Here's how the part is built. I have some questions about the finished solid (model axes, mm). A direction names the side the tool comes from. Round coordinates to 2 decimals unless told otherwise and drop trailing zeros. Order: outer loops, then holes, each group sorted by start corner. A loop starts at its lowest first (then second) coordinate and runs counter-clockwise, first axis right, second up. Notation, with made-up numbers: (88.5, 70) - (119.5, 70) arc R13 ccw to (119.5, 88) - close; hole circle Ø11 at (62.5, -34). An arc over 180 degrees is marked (long way). One line per item, written item: value.
from build123d import *

# Parameters (mm, degrees)
F1_DEPTH    = 63
F2_DEPTH    = 2.5
F3_T        = 4
F3_T3_DEPTH = 132.2533825366
F3_T5_DEPTH = 10.5
F3_T7_DEPTH = 71
F4_W        = 44
F4_H        = 52
F4_W_2      = 45
F5_DEPTH    = 4.5
F7_DEPTH    = 5
F9_DEPTH    = 25


# Not quite as in the source:
# - a shell that OpenCascade refuses in one call is made with other operations: the cavity is built on its own and cut out


with BuildPart() as f1:
    # F0 (on Top) → F1 (new body)
    with BuildSketch(Plane.XY):
        Polygon((26.2132732272, -24.0364130735), (26.2132732272, 29.9635869265), (-65.7867267728, 29.9635869265), (-65.7867267728, -100.0364130735), (26.2132732272, -69.0364130735), align=None)
        Polygon((158.2132732272, 65.9635869265), (26.2132732272, 65.9635869265), (26.2132732272, 29.9635869265), (26.2132732272, -24.0364130735), (26.2132732272, -69.0364130735), (40.4647773284, -64.234275822), (158.2132732272, -24.558152204), align=None)
    extrude(amount=F1_DEPTH)

    # F0 (on Top) → F2 (join)
    with BuildSketch(Plane.XY):
        Polygon((158.2132732272, 65.9635869265), (26.2132732272, 65.9635869265), (26.2132732272, 29.9635869265), (26.2132732272, -24.0364130735), (26.2132732272, -69.0364130735), (40.4647773284, -64.234275822), (158.2132732272, -24.558152204), align=None)
        Polygon((26.2132732272, -24.0364130735), (26.2132732272, 29.9635869265), (-65.7867267728, 29.9635869265), (-65.7867267728, -100.0364130735), (26.2132732272, -69.0364130735), align=None)
        Polygon((158.1303410754, -64.234275822), (158.2132732272, -24.558152204), (40.4647773284, -64.234275822), align=None)
    extrude(amount=F2_DEPTH)

    # F3: shell of thickness 4, made by hand


with BuildPart() as f3_core1:
    # F3_t2: copy of F1
    add(f1.part)

    # the walls: a layer under each face that stays
    f3_faces = [f3_core1.faces().sort_by_distance(p)[0] for p in [
        (46.2132732272, -62.2972826388, 31.5),
        (99.2975592019, -64.234275822, 1.25),
        (158.1718071513, -44.396214013, 1.25),
        (99.3390252778, -57.6215885524, 2.5),
        (158.2132732272, 20.7027173612, 31.5),
        (92.2132732272, 65.9635869265, 31.5),
        (26.2132732272, 47.9635869265, 31.5),
        (-19.7867267728, 29.9635869265, 31.5),
        (46.2132732272, -17.0364130735, 63),
        (-65.7867267728, -35.0364130735, 31.5),
    ]]
    thicken(f3_faces, amount=-F3_T, mode=Mode.SUBTRACT)

    # F3_s4 → F3_t3 (cut)
    with BuildSketch(Plane(origin=(13.1110220732, 4.4178443942, 0), x_dir=(0, 0, 1), z_dir=(0.9476482128, 0.3193162456, 0))):
        Polygon((2.54, 73.8325574618), (2.5, 69.7925574618), (-1.5, 69.7925574618), (-1.5, 73.7925574618), align=None)
    extrude(amount=F3_T3_DEPTH, mode=Mode.SUBTRACT)

    # F3_s6 → F3_t5 (cut)
    with BuildSketch(Plane.XY.offset(-4)):
        Polygon((40.4775499783, -64.3121817506), (39.1875123459, -60.4436829707), (39.8089787227, -60.234275822), (40.4647773284, -60.234275822), align=None)
    extrude(amount=F3_T5_DEPTH, mode=Mode.SUBTRACT)

    # F3_s8 → F3_t7 (cut)
    with BuildSketch(Plane.XY.offset(-4)):
        Polygon((26.1732732272, 30.0035869265), (30.2132732272, 29.9635869265), (30.2132732272, 25.9635869265), (26.2132732272, 25.9635869265), align=None)
    extrude(amount=F3_T7_DEPTH, mode=Mode.SUBTRACT)


with BuildPart() as f1_1:
    add(f1.part)

    # what is left inside the walls is the cavity
    f3_cavity = [f3_core1.part.solids().sort_by_distance(p)[0] for p in [
        (46.213273, -42.323879, 0.04),
    ]]
    add(f3_cavity, mode=Mode.SUBTRACT)

    # F4 (on face) → F5 (cut)
    with BuildSketch(Plane(origin=(-65.7867267728, 0, 0), x_dir=(0, -1, 0), z_dir=(-1, 0, 0))):
        with Locations((68.8298759162, 26)):
            Rectangle(F4_W, F4_H)
        with Locations((3.3298759162, 26)):
            Rectangle(F4_W_2, F4_H)
    extrude(amount=-F5_DEPTH, mode=Mode.SUBTRACT)

    # F6 (on face) → F7 (cut)
    with BuildSketch(Plane.YZ.offset(158.2132732272)):
        Polygon((36.0559523106, 44.5), (-11.5364130735, 44.5), (-11.5364130735, 0), (54.4635869265, 0), (54.4635869265, 44.5), align=None)
    extrude(amount=-F7_DEPTH, mode=Mode.SUBTRACT)

    # F8 (on face) → F9 (cut)
    with BuildSketch(Plane.XY.offset(2.5)):
        with BuildLine():
            ThreePointArc((107.1575140418, -54.484275822), (109.4556110807, -53.5323728609), (110.4075140418, -51.234275822))
            Line((110.4075140418, -51.234275822), (107.1575140418, -51.234275822))
            Line((107.1575140418, -51.234275822), (107.1575140418, -54.484275822))
        make_face()
        with BuildLine():
            Line((107.1575140418, -51.234275822), (110.4075140418, -51.234275822))
            ThreePointArc((110.4075140418, -51.234275822), (104.859417003, -48.9361787832), (107.1575140418, -54.484275822))
            Line((107.1575140418, -54.484275822), (107.1575140418, -51.234275822))
        make_face()
    extrude(amount=-F9_DEPTH, mode=Mode.SUBTRACT)


solid = f1_1.part
Q1. We'd pull the mould along X, two halves only. Please class faces 4 (the flat face through (30.213, 44, 29)), 5 (the flat face through (45, -16, 63)), 6 (the flat face through (26.213, 48, 31)): released by +X, released by -X, zero draft, split by the parting line, or undercut.
Results list:
face 4: undercut
face 5: zero draft
face 6: released by -X
Q2. If we section it at B-B, the plane y = -18: Please give me the cut outline in (x, z).
Results list:
outline: (-65.79, 52) - (-61.79, 52) - (-61.79, 59) - (154.21, 59) - (154.21, 0) - (158.21, 0) - (158.21, 63) - (-65.79, 63) - close
Q3. Which directions (+Z, -Z, +X, -X, +Y, -Y) give clear straight access to the entire face, cutting with the end or side of a thin tool? Please do faces 1 (the flat face through (-19, 29.964, 31)), 2 (the flat face through (125, -53, 2.5)), 3 (the flat face through (93, 61.964, 29)).
Results list:
face 1: +Z, -Z, -X, +Y
face 2: +Z, +X, -Y
face 3: -Z
Q4. If we section it at C-C, the plane z = 9: Please give me the cut outline in (x, y) (3 decimals), then the cut area to 3 significant figures.
Results list:
outline: (-65.787, -100.036) - (158.213, -24.558) - (158.213, -11.536) - (154.213, -11.536) - (154.213, -21.685) - (-61.787, -94.468) - (-61.787, -90.83) - (-65.787, -90.83) - close; (-65.787, -46.83) - (-61.787, -46.83) - (-61.787, -25.83) - (-65.787, -25.83) - close; (-65.787, 19.17) - (-61.787, 19.17) - (-61.787, 25.964) - (30.213, 25.964) - (30.213, 61.964) - (154.213, 61.964) - (154.213, 54.464) - (158.213, 54.464) - (158.213, 65.964) - (26.213, 65.964) - (26.213, 29.964) - (-65.787, 29.964) - close
area: 2,180 mm²
Q5. If I drill on line 1 along X through (y, z) = (48, 48); line 2 along X through (y, z) = (-13, 32); line 3 along Y through (x, z) = (15, 3.5), over which ranges is the centre line in solid material (lowest first)?
Results list:
line 1: 26.21 to 30.21, 154.21 to 158.21
line 2: 154.21 to 158.21
line 3: -72.81 to -68.59, 25.96 to 29.96
Q6. If we section it at D-D, the plane x = 145: Please give me the cut outline in (y, z), then the cut area to 3 significant figures.
Results list:
outline: (-64.23, 0) - (-24.79, 0) - (-24.79, 59) - (61.96, 59) - (61.96, 0) - (65.96, 0) - (65.96, 63) - (-29.01, 63) - (-29.01, 2.5) - (-64.23, 2.5) - close
area: 953 mm²
Q7. Will these pins go through, and if not, where does the flat tip stop? pin 1 (10 mm diameter, centred on x = 135.5, z = 24.5, fed in from -Y); pin 2 (3 mm diameter, centred on x = 156.5, y = 8.5, fed in from -Z); pin 3 (3 mm diameter, centred on x = -26.5, z = 35.5, fed in from +Y).
Results list:
pin 1: y = -33.9
pin 2: z = 44.5
pin 3: y = 29.96
Q8. If we section it at A-A, the plane z = 47.5: Please give me the cut outline in (x, y) (3 decimals), then the cut area to 3 significant figures.
Results list:
outline: (-65.787, -100.036) - (158.213, -24.558) - (158.213, 65.964) - (26.213, 65.964) - (26.213, 29.964) - (-65.787, 29.964) - (-65.787, 19.17) - (-61.787, 19.17) - (-61.787, 25.964) - (30.213, 25.964) - (30.213, 61.964) - (154.213, 61.964) - (154.213, -21.685) - (-61.787, -94.468) - (-61.787, -90.83) - (-65.787, -90.83) - close; (-65.787, -46.83) - (-61.787, -46.83) - (-61.787, -25.83) - (-65.787, -25.83) - close
area: 2,450 mm²
